Check sheet for the modelled part. Datum: model origin and axes. Units: mm. A direction names the side the tool comes from. Coordinates: 2 decimals unless noted, no trailing zeros. Write each loop counter-clockwise with the first axis right and the second up, starting at its lowest first coordinate (ties: lowest second). Pieces come first, ordered by that corner, then holes. Notation, with made-up numbers: (36, -29.5) - (50, -29.5) arc R31 cw to (50, 1.5) - close; hole circle Ø6 at (-8.75, 60.5). An arc over 180 degrees is marked (long way). Answer as CSV lines item,"result". Start each with the question number.
from build123d import *

# Parameters (mm, degrees)
SKETCH1_R            = 18.5
BOSS_EXTRUDE1_DEPTH  = 2
SKETCH2_R            = 17.5
BOSS_EXTRUDE2_DEPTH  = 2
SKETCH3_R            = 6
BOSS_EXTRUDE3_DEPTH  = 5
CUT_EXTRUDE1_REACH   = 29.668
SKETCH4_R            = 3
CUT_EXTRUDE4_DEPTH   = 2
FILLET1_R            = 1
CUT_EXTRUDE5_REACH   = 29.083
SKETCH6_R            = 1.25
FILLET1_OF_MIRROR1_R = 1
CHAMFER1_SIZE        = 1.5
CUT_EXTRUDE6_REACH   = 28.636
SKETCH7_R            = 1.25
CIRPATTERN1_COUNT    = 6
SKETCH9_R            = 1.5
CUT_EXTRUDE7_DEPTH   = 3.5
SKETCH10_R           = 2.75
BOSS_EXTRUDE4_DEPTH  = 6
SKETCH11_R           = 1.25
CUT_EXTRUDE8_DEPTH   = 6
FILLET2_R            = 0.25
CHAMFER2_SIZE        = 0.5
CUT_EXTRUDE9_DEPTH   = 0.3
CIRPATTERN2_COUNT    = 4
CHAMFER3_SIZE        = 0.25


with BuildPart() as part:
    # Sketch1 → Boss-Extrude1 (new body)
    with BuildSketch(Plane(origin=(0, 0, 0), x_dir=(1, 0, 0), z_dir=(0, 1, 0))):
        with Locations(Location((0, 0, 0), (0, 0, 270))):
            Circle(SKETCH1_R)
    extrude(amount=BOSS_EXTRUDE1_DEPTH)

    # Sketch2 → Boss-Extrude2 (add)
    with BuildSketch(Plane(origin=(0, 2, 0), x_dir=(1, 0, 0), z_dir=(0, 1, 0))):
        with Locations(Location((0, 0, 0), (0, 0, 270))):
            Circle(SKETCH2_R)
    extrude(amount=BOSS_EXTRUDE2_DEPTH)

    # Sketch3 → Boss-Extrude3 (add)
    with BuildSketch(Plane.XZ):
        with Locations(Location((0, 0, 0), (0, 0, 90))):
            Circle(SKETCH3_R)
    extrude(amount=BOSS_EXTRUDE3_DEPTH)

    # Sketch4 → Cut-Extrude1 (cut, up to next)
    with BuildSketch(Plane.XZ.offset(5), mode=Mode.PRIVATE) as cut_extrude1_sk1:
        with Locations(Location((0, 0, 0), (0, 0, 270))):
            Circle(SKETCH4_R)
    cut_extrude1_tool1 = extrude(cut_extrude1_sk1.sketch, amount=-CUT_EXTRUDE1_REACH, mode=Mode.PRIVATE) & part.part
    add(cut_extrude1_tool1.solids().sort_by_distance((0, -5, 0))[0], mode=Mode.SUBTRACT)

    # Sketch5 → Cut-Extrude4 (cut)
    with BuildSketch(Plane(origin=(0, 4, 0), x_dir=(1, 0, 0), z_dir=(0, 1, 0))):
        with BuildLine():
            Line((-17.625, 2.625), (-17.625, -2.625))
            Line((-17.625, -2.625), (-15, -2.625))
            ThreePointArc((-15, -2.625), (-12.375, 0), (-15, 2.625))
            Line((-15, 2.625), (-17.625, 2.625))
        make_face()
    cut_extrude4 = extrude(amount=-CUT_EXTRUDE4_DEPTH, mode=Mode.SUBTRACT)

    # Fillet1
    fillet1_edges = [part.edges().sort_by_distance(p)[0] for p in [
        (-17.302004942, 3, -2.625),
        (-17.302004942, 3, 2.625),
    ]]
    fillet(fillet1_edges, radius=FILLET1_R)

    # Sketch6 → Cut-Extrude5 (cut, up to next)
    with BuildSketch(Plane(origin=(0, 2, 0), x_dir=(1, 0, 0), z_dir=(0, 1, 0)), mode=Mode.PRIVATE) as cut_extrude5_sk1:
        with Locations(Location((-15, 0, 0), (0, 0, 270))):
            Circle(SKETCH6_R)
    cut_extrude5_tool1 = extrude(cut_extrude5_sk1.sketch, amount=-CUT_EXTRUDE5_REACH, mode=Mode.PRIVATE) & part.part
    cut_extrude5 = cut_extrude5_tool1.solids().sort_by_distance((-15, 2, 0))[0]
    add(cut_extrude5, mode=Mode.SUBTRACT)

    # Mirror1: Cut-Extrude4, Cut-Extrude5 across plane
    add(cut_extrude4.mirror(Plane(origin=(0, 0, 0), x_dir=(0, 0, 1), z_dir=(1, 0, 0))), mode=Mode.SUBTRACT)
    add(cut_extrude5.mirror(Plane(origin=(0, 0, 0), x_dir=(0, 0, 1), z_dir=(1, 0, 0))), mode=Mode.SUBTRACT)

    # Fillet1 of Mirror1
    fillet1_of_mirror1_edges = [part.edges().sort_by_distance(p)[0] for p in [
        (17.302004942, 3, -2.625),
        (17.302004942, 3, 2.625),
    ]]
    fillet(fillet1_of_mirror1_edges, radius=FILLET1_OF_MIRROR1_R)

    # Chamfer1
    chamfer1_edges = [part.edges().sort_by_distance(p)[0] for p in [
        (-15, 0, -1.25),
        (15, 0, -1.25),
    ]]
    chamfer(chamfer1_edges, length=CHAMFER1_SIZE)

    # Sketch7 → Cut-Extrude6 (cut, up to next)
    with BuildSketch(Plane.XZ, mode=Mode.PRIVATE) as cut_extrude6_sk1:
        with Locations(Location((0, 15, 0), (0, 0, 270))):
            Circle(SKETCH7_R)
    cut_extrude6_tool1 = extrude(cut_extrude6_sk1.sketch, amount=-CUT_EXTRUDE6_REACH, mode=Mode.PRIVATE) & part.part
    cut_extrude6 = cut_extrude6_tool1.solids().sort_by_distance((0, 0, 15))[0]
    add(cut_extrude6, mode=Mode.SUBTRACT)

    # CirPattern1: Cut-Extrude6 ×6 about axis
    cirpattern1_axis = Axis((0, 0, 0), (0, 1, 0))
    for i in range(1, CIRPATTERN1_COUNT):
        add(cut_extrude6.rotate(cirpattern1_axis, i * 360 / CIRPATTERN1_COUNT), mode=Mode.SUBTRACT)

    # Sketch9 → Cut-Extrude7 (cut)
    with BuildSketch(Plane(origin=(0, 4, 0), x_dir=(1, 0, 0), z_dir=(0, 1, 0))):
        with Locations(Location((-5, -8.660254038, 0), (0, 0, 270))):
            Circle(SKETCH9_R)
        with Locations(Location((5, -8.660254038, 0), (0, 0, 270))):
            Circle(SKETCH9_R)
    extrude(amount=-CUT_EXTRUDE7_DEPTH, mode=Mode.SUBTRACT)

    # Sketch10 → Boss-Extrude4 (add)
    with BuildSketch(Plane(origin=(0, 4, 0), x_dir=(1, 0, 0), z_dir=(0, 1, 0))):
        with Locations(Location((-5, 9.797958971, 0), (0, 0, 270))):
            Circle(SKETCH10_R)
        with Locations(Location((5, 9.797958971, 0), (0, 0, 270))):
            Circle(SKETCH10_R)
    extrude(amount=BOSS_EXTRUDE4_DEPTH)

    # Sketch11 → Cut-Extrude8 (cut)
    with BuildSketch(Plane(origin=(0, 10, 0), x_dir=(1, 0, 0), z_dir=(0, 1, 0))):
        with Locations(Location((-5, 9.797958971, 0), (0, 0, 270))):
            Circle(SKETCH11_R)
        with Locations(Location((5, 9.797958971, 0), (0, 0, 270))):
            Circle(SKETCH11_R)
    extrude(amount=-CUT_EXTRUDE8_DEPTH, mode=Mode.SUBTRACT)

    # Fillet2
    fillet2_edges = [part.edges().sort_by_distance(p)[0] for p in [
        (0, 0, -6),
        (0, -5, -6),
    ]]
    fillet(fillet2_edges, radius=FILLET2_R)

    # Chamfer2
    chamfer2_edges = [part.edges().sort_by_distance(p)[0] for p in [
        (0, -5, 3),
    ]]
    chamfer(chamfer2_edges, length=CHAMFER2_SIZE)

    # Sketch12 → Cut-Extrude9 (cut)
    with BuildSketch(Plane.XZ):
        with BuildLine():
            Line((-11.736694594, 1.5), (-8.124038405, 1.5))
            ThreePointArc((-8.124038405, 1.5), (-7.529949879, 1.695600333), (-7.168269181, 2.205882353))
            ThreePointArc((-7.168269181, 2.205882353), (-5.303300859, 5.303300859), (-2.205882353, 7.168269181))
            ThreePointArc((-2.205882353, 7.168269181), (-1.695600333, 7.529949879), (-1.5, 8.124038405))
            Line((-1.5, 8.124038405), (-1.5, 11.736694594))
            ThreePointArc((-1.5, 11.736694594), (-1.87084713, 12.513976182), (-2.708333333, 12.714752477))
            ThreePointArc((-2.708333333, 12.714752477), (-9.192388155, 9.192388155), (-12.714752477, 2.708333333))
            ThreePointArc((-12.714752477, 2.708333333), (-12.513976182, 1.87084713), (-11.736694594, 1.5))
        make_face()
    cut_extrude9 = extrude(amount=-CUT_EXTRUDE9_DEPTH, mode=Mode.SUBTRACT)

    # CirPattern2: Cut-Extrude9 ×4 about axis
    cirpattern2_axis = Axis((0, 0, 0), (0, 1, 0))
    for i in range(1, CIRPATTERN2_COUNT):
        add(cut_extrude9.rotate(cirpattern2_axis, i * 360 / CIRPATTERN2_COUNT), mode=Mode.SUBTRACT)

    # Chamfer3
    chamfer3_edges = [part.edges().sort_by_distance(p)[0] for p in [
        (0, 0, 16.25),
        (14.072912811, 0, 8.125),
        (14.072912811, 0, -8.125),
        (0, 0, -16.25),
        (-14.072912811, 0, -8.125),
        (-14.072912811, 0, 8.125),
    ]]
    chamfer(chamfer3_edges, length=CHAMFER3_SIZE)


solid = part.part
(1) Cross-section at A-A on y = 4.5. Record the boundary of the cut face in (x, z), plus the area to 3 significant figures.
(2) Tool access check on faces 5 (the face through (-0.331, 2.986, 17.497)), 6 (the face through (-8, 0, 0)), 7 (the face through (-5, 4, -10)). Record the directions out of +Z, -Z, +X, -X, +Y, -Y that give a thin tool (end or side, any length) a straight path to the whole face; none if there is none.
(3) Material ranges on probe 1 along X at (y, z) = (1.8, 0); probe 2 along Z at (x, y) = (-9, 0.25); probe 3 along Y at (x, z) = (-2, -6.5), recorded low to high. Write a range as from..to.
(4) Release check for a two-part mould opening along Z. For faces 1 (the face through (6.265, 2.274, 9.467)), 2 (the face through (0, 4, 4)), 3 (the face through (0.331, 2.986, -17.497)), 4 (the face through (-14.23, 2.1, 7.34)) record: pulls with the +Z half, pulls with the -Z half, needs draft (parallel to the pull), parting line crosses it, or undercut.
(5) Go/stop test with flat-tipped pins: P1, Ø1, axis at x = -14, z = -9.5, coming from the -Y side; P2, Ø8, axis at x = 0, y = 7.5, coming from the -Z side; P3, Ø0.9, axis at x = -5.5, z = 9, coming from the +Y side; P4, Ø12.5, axis at x = -6.5, z = 7.5, coming from the -Y side. Record where each tip stops, or that it passes through.
(6) Cross-section at D-D on z = -15. Record the boundary of the cut face in (x, y).
(7) Cross-section at B-B on z = 0. State how many separate pieces and enclosed holes the cut face has, plus the area to 3 significant figures.
Checked values:
1,outline,"circle Ø5.5 at (-5, -9.8); circle Ø5.5 at (5, -9.8); hole circle Ø2.5 at (-5, -9.8); hole circle Ø2.5 at (5, -9.8)"
1,area,"37.7 mm^2"
2,face 5,"+Z, +Y"
2,face 6,"-Y"
2,face 7,"+Y"
3,probe 1,"-18.5..-16.25, -13.75..-3, 3..13.75, 16.25..18.5"
3,probe 2,"-16.16..-9.38, -1.5..1.5, 9.38..16.16"
3,probe 3,"0..4"
4,face 1,"undercut"
4,face 2,"needs draft"
4,face 3,"pulls with the -Z half"
4,face 4,"undercut"
5,P1,"y = 0"
5,P2,"z = -17.5"
5,P3,"y = 0.5"
5,P4,"y = -5"
6,outline,"(-10.83, 0) - (-1.5, 0) - (-1.25, 0.25) - (-1.25, 4) - (-9.01, 4) - (-9.01, 2) - (-10.83, 2) - close; (1.25, 0.25) - (1.5, 0) - (10.83, 0) - (10.83, 2) - (9.01, 2) - (9.01, 4) - (1.25, 4) - close"
7,separate pieces,"4"
7,enclosed holes,"0"
7,area,"115 mm^2"
